from build123d import *

# Parameters (mm, degrees)
SKETCH1_R           = 6
BOSS_EXTRUDE1_DEPTH = 15
SKETCH2_R           = 2.6
CUT_EXTRUDE1_DEPTH  = 10
SKETCH5_W           = 3.25
SKETCH5_H           = 3.25
CUT_EXTRUDE2_DEPTH  = 5
CHAMFER1_SIZE       = 0.5


with BuildPart() as part:
    # Sketch1 → Boss-Extrude1 (new body)
    with BuildSketch(Plane.XY):
        Circle(SKETCH1_R)
    extrude(amount=BOSS_EXTRUDE1_DEPTH)

    # Sketch2 → Cut-Extrude1 (cut)
    with BuildSketch(Plane(origin=(0, 0, 0), x_dir=(-1, 0, 0), z_dir=(0, 0, -1))):
        Circle(SKETCH2_R)
    extrude(amount=-CUT_EXTRUDE1_DEPTH, mode=Mode.SUBTRACT)

    # Sketch5 → Cut-Extrude2 (cut)
    with BuildSketch(Plane.XY.offset(15)):
        Rectangle(SKETCH5_W, SKETCH5_H)
    extrude(amount=-CUT_EXTRUDE2_DEPTH, mode=Mode.SUBTRACT)

    # Chamfer1
    chamfer1_edges = [part.edges().sort_by_distance(p)[0] for p in [
        (1.625, 0, 15),
        (0, 1.625, 15),
        (-1.625, 0, 15),
        (0, -1.625, 15),
        (2.6, 0, 0),
    ]]
    chamfer(chamfer1_edges, length=CHAMFER1_SIZE)


solid = part.part
For this review, take the finished solid that the model builds, in its own axes (mm). A direction names the side the tool comes from. Give positions to 0.01 mm unless a question says otherwise; leave off trailing zeros. Loops run counter-clockwise (first coordinate to the right, second up) from the corner with the lowest first, then second, coordinate; pieces in that order, holes last. Notation, with made-up numbers: M 3.25,88.5 L 21.25,88.5 A4 ccw 21.25,95.5 Z; hole C 61.25,83 d2. An arc over 180 degrees is marked long. Answer as a JSON object with one key per item and string values. Group by question number.
Q1. Add section D-D on y = 3.5. Give the boundary of the cut face in (x, z), and give its area (3 significant figures).
Q2. Add section A-A on y = 0. Give the boundary of the cut face in (x, z) (3 decimals), and give its area (3 significant figures).
Q3. Tool access review of faces 1 (the flat face through (-2, 0, 10)), 2 (the flat face through (3, -3, 0)), 3 (the flat face through (0, -1.625, 12)): name each direction out of +Z, -Z, +X, -X, +Y, -Y from which nothing blocks a thin tool from reaching the whole face with its end or side.
Q4. Mouldability with a two-part tool opening along Y and no side actions: class faces 4 (the cylindrical face through (-6, 0, 7)), 5 (the flat face through (3, 0, 15)), 6 (the flat face through (0, 1.625, 12)) as +Y half, -Y half, draft (parallel to the pull), parting line (faces both ways), or undercut.
Q5. Add section C-C on z = 6. Give the boundary of the cut face in (x, y).
Q6. Insertion check: P1, Ø1.5, axis at y = -4, z = 8, coming from the -X side; P2, Ø1, axis at x = -3.5, z = 4.5, coming from the -Y side; P3, Ø1, axis at x = -1.5, z = 3.5, coming from the +Y side. Each pin has a flat end and moves straight along its axis. Give the tip position at first contact, or say it passes through.
Q7. For probe 1 along Y at (x, z) = (0, 5.75); probe 2 along Y at (x, z) = (-1, 1.25); probe 3 along Z at (x, y) = (-0.5, -2.5), list the stretches that pass through material, from the lowest coordinate up. Write a range as [from, to].
Checked values:
{
 "1": {"outline": "M -4.87,0 L 4.87,0 L 4.87,15 L -4.87,15 Z", "area": "146 mm²"},
 "2": {"outline": "M -6,0 L -3.1,0 L -2.6,0.5 L -2.6,10 L -1.625,10 L -1.625,14.5 L -2.125,15 L -6,15 Z; M 1.625,10 L 2.6,10 L 2.6,0.5 L 3.1,0 L 6,0 L 6,15 L 2.125,15 L 1.625,14.5 Z", "area": "111 mm²"},
 "3": {"face 1": "-Z", "face 2": "-Z, +X, -X, +Y, -Y", "face 3": "+Z, -Z"},
 "4": {"face 4": "parting line", "face 5": "draft", "face 6": "undercut"},
 "5": {"outline": "C 0,0 d12; hole C 0,0 d5.2"},
 "6": {"P1": "x = -5.04", "P2": "y = -5.2", "P3": "y = 5.92"},
 "7": {"probe 1": "[-6, -2.6], [2.6, 6]", "probe 2": "[-5.92, -2.4], [2.4, 5.92]", "probe 3": "[10, 15]"}
}
